Verification items for the finished model (mm, model axes). Give positions to 0.01 mm unless a question says otherwise; leave off trailing zeros. Write each loop counter-clockwise with the first axis right and the second up, starting at its lowest first coordinate (ties: lowest second). Pieces come first, ordered by that corner, then holes. Notation, with made-up numbers: (65, 33) - (120, 33) arc R20 cw to (120, 57) - close; hole circle Ø9 at (71.25, 64.5). An arc over 180 degrees is marked (long way). Answer as a JSON object with one key per item and string values. Group by question number.
Item 1: Sectioned sample at D-D, the plane y = 169. Record the boundary of the cut face in (x, z), and give its area (3 significant figures).
Item 2: Sectioned sample at B-B, the plane y = 114.3. Record the boundary of the cut face in (x, z), and give its area (3 significant figures).
Item 3: Draft check along Y on faces 1 (the face through (-333, 184.15, -29)), 2 (the face through (-252, -25.4, -14)), 3 (the face through (-91.584, 8.005, 3.219)). Enter one of: +Y half, -Y half, draft (parallel to the pull), parting line (faces both ways), or undercut.
Item 4: Go/stop test with flat-tipped pins: pin 1 (1.5 mm diameter, centred on x = -174.5, y = 53, fed in from -Z); pin 2 (10 mm diameter, centred on x = -285.5, z = -15.5, fed in from -Y); pin 3 (4 mm diameter, centred on x = -322.5, y = 107.5, fed in from +Z); pin 4 (21.5 mm diameter, centred on x = -109, z = -5, fed in from +Y). Record where each tip stops, or that it passes through.
Item 5: Sectioned sample at A-A, the plane x = -44.45. Record the boundary of the cut face in (y, z).
Item 6: Sectioned sample at C-C, the plane x = -353. Record the boundary of the cut face in (y, z).
Item 7: Scan lines: line 1 along Y through (x, z) = (-44.45, 4.25); line 2 along Y through (x, z) = (-19, 3); line 3 along Z through (x, y) = (-97, 42.5). Record each from-to range of solid material in increasing order. Write a range as [from, to].
```python
from build123d import *

# Parameters (mm, degrees)
F1_DEPTH = 152.4
F2_R     = 7.14375
F3_DEPTH = 63.5931574972
F4_R     = 3.96875
F5_DEPTH = 37.70193717
F7_DEPTH = 6.35
F8_R     = 4.365625
F8_W     = 105.4455175215
F8_H     = 1.5875
F9_DEPTH = 72.8023226846


with BuildPart() as f1:
    # F0 (on Front) → F1 (new body)
    with BuildSketch(Plane.XZ):
        Polygon((-152.4, 0), (0, 0), (0, 6.35), (-152.4, 6.35), (-331.2859139551, -25.192413099), (-330.2, -31.35093717), align=None)
    extrude(amount=-F1_DEPTH)

    # F2 (on face) → F3 (cut, through all)
    with BuildSketch(Plane(origin=(-5.6813362512, 0, 32.2204589924), x_dir=(0.984807753, 0, 0.1736481777), z_dir=(-0.1736481777, 0, 0.984807753))):
        with Locations((-278.2400531523, 76.2)):
            Circle(F2_R)
    extrude(amount=-F3_DEPTH, mode=Mode.SUBTRACT)

    # F4 (on face) → F5 (cut, through all)
    with BuildSketch(Plane.XY.offset(6.35)):
        with Locations((-19.05, 127)):
            Circle(F4_R)
        with Locations((-19.05, 25.4)):
            Circle(F4_R)
        with Locations((-88.9, 25.4)):
            Circle(F4_R)
        with Locations((-88.9, 127)):
            Circle(F4_R)
        with Locations((-95.25, 9.525)):
            Circle(F4_R)
        with Locations((-95.25, 142.875)):
            Circle(F4_R)
        with Locations((-68.2625, 114.3)):
            Circle(F4_R)
        with Locations((-44.45, 114.3)):
            Circle(F4_R)
        with Locations((-68.2625, 38.1)):
            Circle(F4_R)
        with Locations((-44.45, 38.1)):
            Circle(F4_R)
    extrude(amount=-F5_DEPTH, mode=Mode.SUBTRACT)

    # F6 (on face) → F7 (join)
    with BuildSketch(Plane(origin=(-5.6813362512, 0, 32.2204589924), x_dir=(0.984807753, 0, 0.1736481777), z_dir=(-0.1736481777, 0, 0.984807753))):
        Polygon((-330.6275531523, 120.65), (-330.6275531523, 152.4), (-225.1820356309, 152.4), (-225.1820356309, 177.8), (-275.9820356309, 177.8), (-282.3320356309, 184.15), (-383.9320356309, 184.15), (-383.9320356309, 120.65), align=None)
        Polygon((-383.9320356309, -31.75), (-282.3320356309, -31.75), (-275.9820356309, -25.4), (-225.1820356309, -25.4), (-225.1820356309, 0), (-330.6275531523, 0), (-330.6275531523, 31.75), (-383.9320356309, 31.75), align=None)
    extrude(amount=-F7_DEPTH)

    # F8 (on face) → F9 (cut, through all)
    with BuildSketch(Plane(origin=(-5.6813362512, 0, 32.2204589924), x_dir=(0.984807753, 0, 0.1736481777), z_dir=(-0.1736481777, 0, 0.984807753))):
        with Locations((-368.0570356309, 133.35)):
            Circle(F8_R)
        with Locations((-368.0570356309, 19.05)):
            Circle(F8_R)
        with Locations((-277.9047943916, 119.85625)):
            Rectangle(F8_W, F8_H)
        with Locations((-277.9047943916, 32.54375)):
            Rectangle(F8_W, F8_H)
    extrude(amount=-F9_DEPTH, mode=Mode.SUBTRACT)


solid = f1.part
```
Geometry check:
{
 "1": {"outline": "(-383.78, -34.45) - (-382.68, -40.7) - (-226.34, -13.14) - (-227.44, -6.88) - close", "area": "1,010 mm^2"},
 "2": {"outline": "(-331.29, -25.19) - (-330.2, -31.35) - (-152.4, 0) - (-72.23, 0) - (-72.23, 6.35) - (-152.4, 6.35) - close; (-64.29, 0) - (-48.42, 0) - (-48.42, 6.35) - (-64.29, 6.35) - close; (-40.48, 0) - (0, 0) - (0, 6.35) - (-40.48, 6.35) - close", "area": "2,000 mm^2"},
 "3": {"face 1": "+Y half", "face 2": "-Y half", "face 3": "undercut"},
 "4": {"pin 1": "z = -4.03", "pin 2": "y = -31.75", "pin 3": "z = -23.29", "pin 4": "y = 152.4"},
 "5": {"outline": "(0, 0) - (34.13, 0) - (34.13, 6.35) - (0, 6.35) - close; (42.07, 0) - (110.33, 0) - (110.33, 6.35) - (42.07, 6.35) - close; (118.27, 0) - (152.4, 0) - (152.4, 6.35) - (118.27, 6.35) - close"},
 "6": {"outline": "(-31.75, -35.47) - (31.75, -35.47) - (31.75, -29.02) - (-31.75, -29.02) - close; (120.65, -35.47) - (184.15, -35.47) - (184.15, -29.02) - (120.65, -29.02) - close"},
 "7": {"line 1": "[0, 34.13], [42.07, 110.33], [118.27, 152.4]", "line 2": "[0, 21.43], [29.37, 123.03], [130.97, 152.4]", "line 3": "[0, 6.35]"}
}
